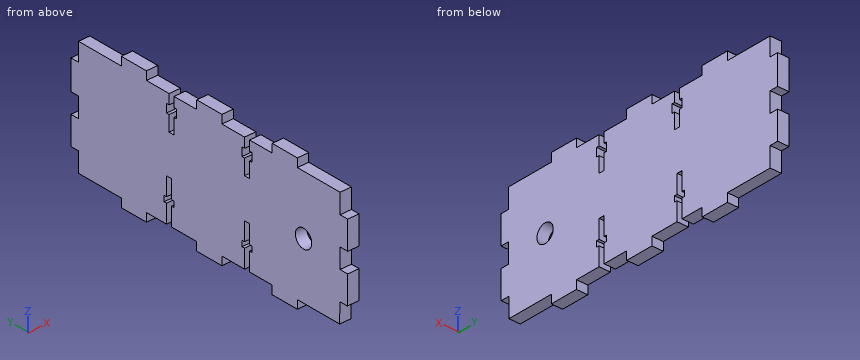
from build123d import *

# Parameters (mm, degrees)
F0_R     = 3.25
F1_DEPTH = 4.064


with BuildPart() as f1:
    # F0 (on Right) → F1 (new body)
    with BuildSketch(Plane.YZ):
        Polygon((-47.118501, 17.030547), (-50.118501, 17.030547), (-50.118501, 7.030547), (-47.118501, 7.030547), (-47.118501, 0.030547), (-50.118346, 0), (-50.016524, -9.999482), (-47.016679, -9.968935), (-46.945404, -16.968572), (-30.118501, -16.968572), (-30.118501, -19.968572), (-20.118501, -19.968572), (-20.118501, -16.968572), (-11.118501, -16.968572), (-11.118501, -10.468572), (-12.118501, -10.468572), (-12.118501, -8.468572), (-11.118501, -8.468572), (-11.118501, -1.968572), (-9.118501, -1.968572), (-9.118501, -8.468572), (-8.118501, -8.468572), (-8.118501, -10.468572), (-9.118501, -10.468572), (-9.118501, -16.968572), (-0.118501, -16.968572), (-0.118501, -19.968572), (9.881499, -19.968572), (9.881499, -16.968572), (19.881499, -16.968572), (19.881499, -10.468572), (18.881499, -10.468572), (18.881499, -8.468572), (19.881499, -8.468572), (19.881499, -1.968572), (21.881499, -1.968572), (21.881499, -8.468572), (22.881499, -8.468572), (22.881499, -10.468572), (21.881499, -10.468572), (21.881499, -16.968572), (29.881499, -16.968572), (29.881499, -19.968572), (39.881499, -19.968572), (39.881499, -16.968572), (56.881499, -16.968572), (56.881499, -9.999482), (59.881499, -9.999482), (59.881499, 0), (56.881499, 0), (56.881499, 7.030547), (59.881499, 7.030547), (59.881499, 17.530547), (56.881499, 17.530547), (56.881499, 24.030547), (39.881499, 24.030547), (39.881499, 27.030547), (29.881499, 27.030547), (29.881499, 24.030547), (20.881499, 24.030547), (20.881499, 20.530547), (21.881499, 20.530547), (21.881499, 17.530547), (20.881499, 17.530547), (20.881499, 12.030547), (18.881499, 12.030547), (18.881499, 17.530547), (17.881499, 17.530547), (17.881499, 20.530547), (18.881499, 20.530547), (18.881499, 24.030547), (9.881499, 24.030547), (9.881499, 27.030547), (-0.118501, 27.030547), (-0.118501, 24.030547), (-9.118501, 24.030547), (-9.118501, 20.530547), (-8.118501, 20.530547), (-8.118501, 17.530547), (-9.118501, 17.530547), (-9.118501, 12.030547), (-11.118501, 12.030547), (-11.118501, 17.530547), (-12.118501, 17.530547), (-12.118501, 20.530547), (-11.118501, 20.530547), (-11.118501, 24.030547), (-20.118501, 24.030547), (-20.118501, 27.030547), (-30.118501, 27.030547), (-30.118501, 24.030547), (-47.118501, 24.030547), align=None)
        with Locations((-32.581907, 3.088805)):
            Circle(F0_R, mode=Mode.SUBTRACT)
    extrude(amount=F1_DEPTH)


solid = f1.part
Could you check a few things on this model? Use its own coordinates, in mm. Round coordinates to 2 decimals unless told otherwise and drop trailing zeros. Loops run counter-clockwise (first coordinate to the right, second up) from the corner with the lowest first, then second, coordinate; pieces in that order, holes last. Notation, with made-up numbers: (-8.75, -32) - (10.25, -32) arc R21 cw to (10.25, -11) - close; hole circle Ø7 at (-29, 78.25). An arc over 180 degrees is marked (long way). Write item = value, one per line.
1) Imagine slicing it at C-C (y = -17). Please give me the cut outline in (x, z).
Computed:
outline = (0, -16.97) - (4.06, -16.97) - (4.06, 24.03) - (0, 24.03) - close
2) I'm going to push flat-ended pins straight in: P1, Ø1.5, axis at x = 2.5, z = 26, coming from the -Y side; P2, Ø2, axis at x = 1, y = 52, coming from the -Z side; P3, Ø1.8, axis at x = 1.5, z = 22, coming from the +Y side. Where does each tip first touch, or does it pass through?
Computed:
P1 = -30.12
P2 = -16.97
P3 = 56.88
3) I need wall thicknesses on line 1 along Y through (x, z) = (2.25, 19); line 2 along Y through (x, z) = (1.8, 21); line 3 along Z through (x, y) = (0.3, -31). Which ranges of each line are inside material? Lowest first, please. Write a range as from..to.
Computed:
line_1 = -47.12..-12.12, -8.12..17.88, 21.88..56.88
line_2 = -47.12..-11.12, -9.12..18.88, 20.88..56.88
line_3 = -16.97..0.25, 5.93..24.03
4) Imagine slicing it at B-B (z = 5). Please give me the cut outline in (x, y), and give its area (3 significant figures).
Computed:
outline = (0, -47.12) - (4.06, -47.12) - (4.06, -35.21) - (0, -35.21) - close; (0, -29.95) - (4.06, -29.95) - (4.06, 56.88) - (0, 56.88) - close
area = 401 mm2
5) Imagine slicing it at A-A (z = 13.5). Please give me the cut outline in (x, y).
Computed:
outline = (0, -50.12) - (4.06, -50.12) - (4.06, -11.12) - (0, -11.12) - close; (0, -9.12) - (4.06, -9.12) - (4.06, 18.88) - (0, 18.88) - close; (0, 20.88) - (4.06, 20.88) - (4.06, 59.88) - (0, 59.88) - close
